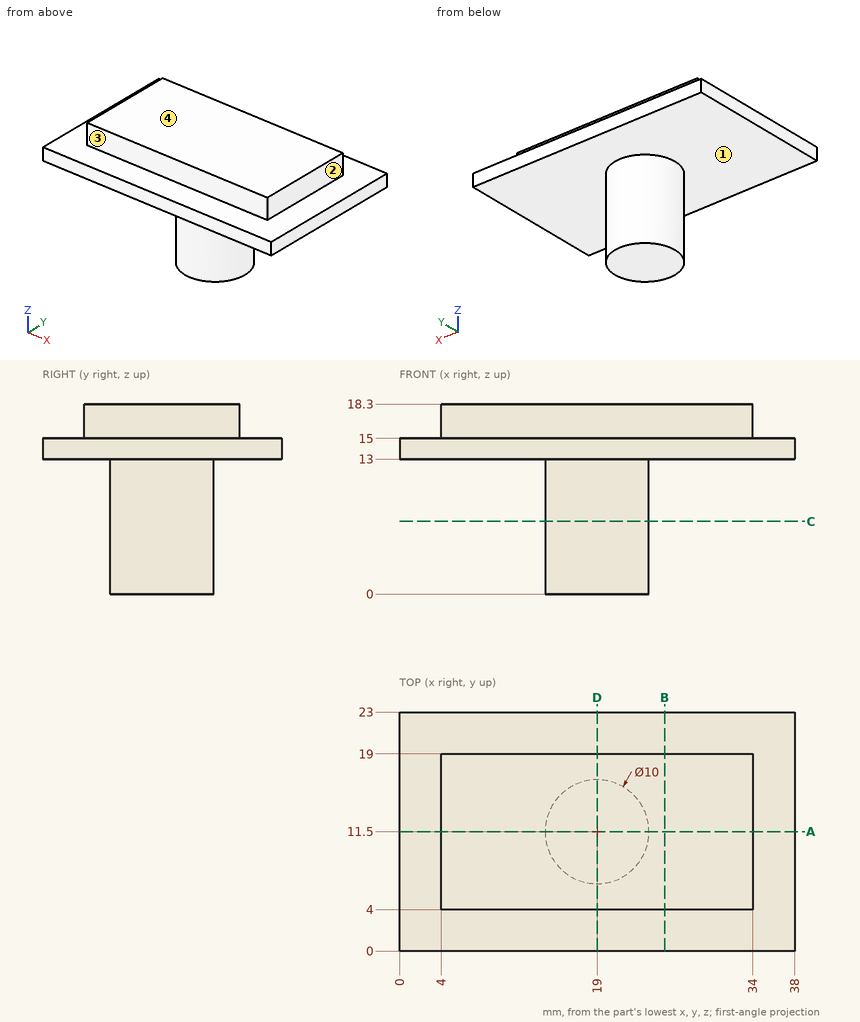
Source: three-view drawing plus pictorial views. Frame: mm from the lowest corner of the part. A direction names the side the tool comes from. Coordinates: 2 decimals unless noted, no trailing zeros. Loops run counter-clockwise (first coordinate to the right, second up) from the corner with the lowest first, then second, coordinate; pieces in that order, holes last. Notation, with made-up numbers: (-17, 84) - (10, 84) arc R24 ccw to (10, 104) - close; hole circle Ø4 at (56, 11.5). An arc over 180 degrees is marked (long way). Answer in a Markdown table with one row per item. Add a question column.
Item 1: Section query C-C on z = 7. Return the cut outline in (x, y).
Item 2: Contact query for flat-ended pins moving along their axis: P1, Ø1, axis at x = 18.5, z = 8, coming from the -Y side; P2, Ø1.7, axis at y = 9.5, z = 16, coming from the +X side; P3, Ø1.5, axis at x = 23.5, z = 8.5, coming from the +Y side. Output: stop coordinate, or through.
Item 3: Access query for the marked faces 1, 2, 3 and 4. Directions: +Z, -Z, +X, -X, +Y, -Y. A direction counts if a zero-diameter tool reaches every point of the face in a straight line with its end or side. Return the directions, or none.
Item 4: Section query B-B on x = 25.5. Return the cut outline in (y, z), then the cut area to 3 significant figures.
Item 5: Section query D-D on x = 19. Return the cut outline in (y, z), then the cut area to 4 significant figures.
Item 6: Line query: line 1 along Z through (x, y) = (2.5, 9); line 2 along Z through (x, y) = (11.5, 10); line 3 along Y through (x, z) = (8, 16.25). Output: solid intervals per line, ascending. Write a range as [from, to].
Item 7: Section query A-A on y = 11.5. Return the cut outline in (x, z).
Recorded:
| question | item | result |
|---|---|---|
| 1 | outline | circle Ø10 at (19, 11.5) |
| 2 | P1 | y = 6.5 |
| 2 | P2 | x = 34 |
| 2 | P3 | y = 14.81 |
| 3 | face 1 | -Z |
| 3 | face 2 | +Z, +X, +Y, -Y |
| 3 | face 3 | +Z, +X, -X, -Y |
| 3 | face 4 | +Z, +X, -X, +Y, -Y |
| 4 | outline | (0, 13) - (23, 13) - (23, 15) - (19, 15) - (19, 18.3) - (4, 18.3) - (4, 15) - (0, 15) - close |
| 4 | area | 95.5 mm^2 |
| 5 | outline | (0, 13) - (6.5, 13) - (6.5, 0) - (16.5, 0) - (16.5, 13) - (23, 13) - (23, 15) - (19, 15) - (19, 18.3) - (4, 18.3) - (4, 15) - (0, 15) - close |
| 5 | area | 225.5 mm^2 |
| 6 | line 1 | [13, 15] |
| 6 | line 2 | [13, 18.3] |
| 6 | line 3 | [4, 19] |
| 7 | outline | (0, 13) - (14, 13) - (14, 0) - (24, 0) - (24, 13) - (38, 13) - (38, 15) - (34, 15) - (34, 18.3) - (4, 18.3) - (4, 15) - (0, 15) - close |
